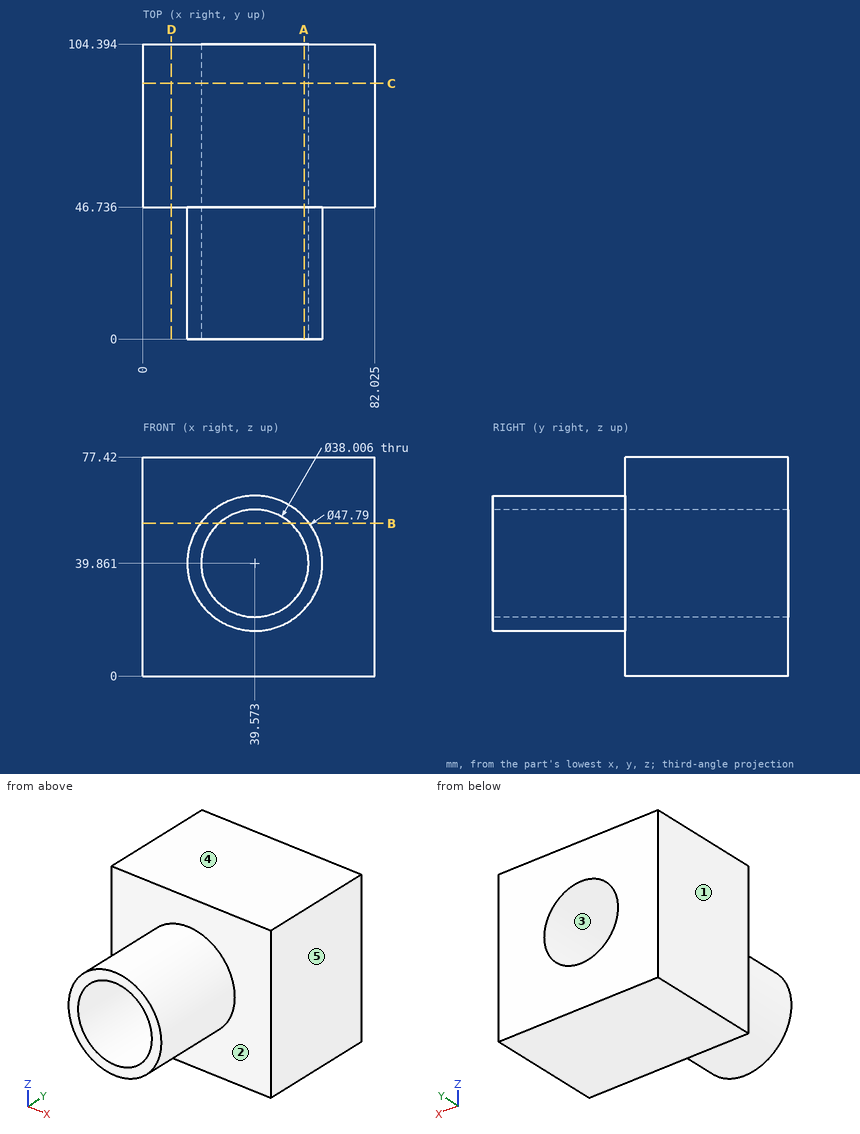
Here's the drawing with two shaded views (mm, measured from the low corner). I have some questions. A direction names the side the tool comes from. Coordinates: 2 decimals unless noted, no trailing zeros. Order: outer loops, then holes, each group sorted by start corner. A loop starts at its lowest first (then second) coordinate and runs counter-clockwise, first axis right, second up.
Item 1: If we section it at C-C, the plane y = 90.5: List the corners of the cut face in (x, z) for me (1 decimal), then the cut area to 3 significant figures.
Response values:
outline: (0, 0) - (82, 0) - (82, 77.4) - (0, 77.4) - close; hole circle Ø38 at (39.6, 39.9)
area: 5,220 mm2
Item 2: I need wall thicknesses on probe 1 along Y at (x, z) = (71, 46); probe 2 along Z at (x, y) = (44.5, 98) (1 decimal); probe 3 along X at (y, z) = (54.5, 29) (1 decimal). Which ranges of each line are inside material? Lowest first, please.
Response values:
probe 1: y = 46.74 to 104.39
probe 2: z = 0 to 21.5, 58.2 to 77.4
probe 3: x = 0 to 24, 55.2 to 82
Item 3: I'm going to push flat-ended pins straight in: pin 1 Ø3 at (y, z) = (30, 30.5) entering from +X; pin 2 Ø23 at (x, z) = (39.57, 39.86) entering from +Y; pin 3 Ø12 at (y, z) = (40.5, 58) entering from +X (1 decimal); pin 4 Ø10 at (x, z) = (72, 13) entering from -Y. Where does each tip first touch, or does it pass through?
Response values:
pin 1: stops at x = 62.14
pin 2: passes through
pin 3: stops at x = 60.2
pin 4: stops at y = 46.74
Item 4: If we section it at B-B, the plane z = 54: List the corners of the cut face in (x, y) for me (1 decimal).
Response values:
outline: (0, 46.7) - (20.3, 46.7) - (20.3, 0) - (26.9, 0) - (26.9, 104.4) - (0, 104.4) - close; (52.3, 0) - (58.8, 0) - (58.8, 46.7) - (82, 46.7) - (82, 104.4) - (52.3, 104.4) - close
Item 5: If we section it at A-A, the plane x = 57: List the corners of the cut face in (y, z) for me.
Response values:
outline: (0, 23.51) - (46.74, 23.51) - (46.74, 0) - (104.39, 0) - (104.39, 32.28) - (0, 32.28) - close; (0, 47.44) - (104.39, 47.44) - (104.39, 77.42) - (46.74, 77.42) - (46.74, 56.21) - (0, 56.21) - close
Item 6: If we section it at D-D, the plane x = 10: List the corners of the cut face in (y, z) for me, then the cut area to 3 significant figures.
Response values:
outline: (46.74, 0) - (104.39, 0) - (104.39, 77.42) - (46.74, 77.42) - close
area: 4,460 mm2
Item 7: Thinking about a two-plate mould opening in Z: for the marked faces 3, 4 and 5, which applies, pulls with the +Z half, pulls with the -Z half, needs draft (parallel to the pull), parting line crosses it, or undercut?
Response values:
face 3: undercut
face 4: pulls with the +Z half
face 5: needs draft
Item 8: Which directions (+Z, -Z, +X, -X, +Y, -Y) give clear straight access to the entire face, cutting with the end or side of a thin tool? Please do the marked faces 1 and 2.
Response values:
face 1: +Z, -Z, -X, +Y, -Y
face 2: -Y
